from build123d import *

# Parameters (mm, degrees)
SKETCH_1_W               = 50
SKETCH_1_H               = 60
EXTRUDE_1_DEPTH          = 70
DRAFT_1_ANGLE            = 1.591
CUT_EXTRUDE_1_DEPTH      = 105.880884817
CUT_EXTRUDE_1_DEPTH_BACK = 105.880884817
SKETCH_8_R               = 30
SKETCH_9_R               = 29.988439116
CUT_EXTRUDE_2_DEPTH      = 93.836652593
SKETCH_10_W              = 61.388766385
SKETCH_10_H              = 50
CUT_EXTRUDE_3_DEPTH      = 93.836652759
SHELL_1_T                = -3
SKETCH_11_R              = 2.125
CUT_EXTRUDE_4_DEPTH      = 64.305956024


with BuildPart() as part:
    # 草圖1 → 填料-伸長1 (new body)
    with BuildSketch(Plane(origin=(0, 0, 0), x_dir=(1, 0, 0), z_dir=(0, 1, 0))):
        with Locations((25, 0)):
            Rectangle(SKETCH_1_W, SKETCH_1_H)
    extrude(amount=EXTRUDE_1_DEPTH)

    # 拔模1
    draft_1_faces = [part.faces().sort_by_distance(p)[0] for p in [
        (50, 35, 0),
        (25, 35, -30),
    ]]
    draft(draft_1_faces, Plane.ZX.offset(70), DRAFT_1_ANGLE)

    # 草圖8 → 除料-伸長1 (cut, two sides: drawn at the far end of the back side and taken through both)
    with BuildSketch(Plane(origin=(50, 70, -30), x_dir=(0.9996147856379402, 0.027743225206125616, 0.0007705771714084014), z_dir=(0.027753924659674706, -0.9992294227713525, -0.027753924659674706)).offset(-CUT_EXTRUDE_1_DEPTH_BACK)):
        Circle(SKETCH_8_R)
    extrude(amount=CUT_EXTRUDE_1_DEPTH + CUT_EXTRUDE_1_DEPTH_BACK, mode=Mode.SUBTRACT)

    # 草圖9 → 除料-伸長2 (cut, through all)
    with BuildSketch(Plane(origin=(0, 70, 0), x_dir=(1, 0, 0), z_dir=(0, 1, 0))):
        with Locations((50, -30)):
            Circle(SKETCH_9_R)
    extrude(amount=-CUT_EXTRUDE_2_DEPTH, mode=Mode.SUBTRACT)

    # 草圖10 → 除料-伸長3 (cut, through all)
    with BuildSketch(Plane.ZY):
        with Locations((-0.694383192, 45)):
            Rectangle(SKETCH_10_W, SKETCH_10_H)
    extrude(amount=-CUT_EXTRUDE_3_DEPTH, mode=Mode.SUBTRACT)

    # 薄殼1
    shell_1_openings = [part.faces().sort_by_distance(p)[0] for p in [
        (14.872442298, 20, -1.069608967),
        (10.828073147, 9.957245624, -31.667707178),
        (10.005780442, 10, 30),
        (0, 9.984986274, -0.833468336),
    ]]
    offset(amount=SHELL_1_T, openings=shell_1_openings, kind=Kind.INTERSECTION)

    # 草圖11 → 除料-伸長4 (cut, through all)
    with BuildSketch(Plane(origin=(0, 3, 0), x_dir=(1, 0, 0), z_dir=(0, 1, 0))):
        with Locations(Location((10, 15, 0), (0, 0, 270))):
            Circle(SKETCH_11_R)
        with Locations(Location((10, -15, 0), (0, 0, 90))):
            Circle(SKETCH_11_R)
    extrude(amount=-CUT_EXTRUDE_4_DEPTH, mode=Mode.SUBTRACT)


solid = part.part
Source: CAD feature listing. Evaluate the final solid. Frame: model axes, mm. Give positions to 0.01 mm unless a question says otherwise; leave off trailing zeros. Write each loop counter-clockwise with the first axis right and the second up, starting at its lowest first coordinate (ties: lowest second). Pieces come first, ordered by that corner, then holes. Notation, with made-up numbers: M 59,52.25 L 91,52.25 A15 ccw 91,73.25 Z; hole C 84.25,26.5 d5. An arc over 180 degrees is marked long. Return JSON: item names as keys, results as strings. Group by question number.
1) Cut plane A-A, the plane x = 10. Output: boundary loops of the cut face in (y, z) (3 decimals), plus the area to 3 significant figures.
2) Material intervals for line 1 along Y through (x, z) = (15, -8); line 2 along X through (y, z) = (1.2, 15) (3 decimals); line 3 along Z through (x, y) = (38.5, 10), sorted ascending. Write a range as [from, to].
3) Pull-direction query (X, two-part tool) for faces 1 (the face through (0, 1, -1)), 2 (the face through (11, 3, -1)), 3 (the face through (11.29, 1.52, 16.69)); classes: pulls with the +X half, pulls with the -X half, needs draft (parallel to the pull), parting line crosses it, or undercut.
4) Cut plane B-B, the plane z = 15.5. Output: boundary loops of the cut face in (x, y), plus the area to 3 significant figures.
5) Pin query (flat end, axial travel): P1, Ø5, axis at x = 10, z = 15, coming from the +Y side; P2, Ø6, axis at y = 9, z = -20.5, coming from the +X side; P3, Ø5, axis at y = 11, z = -18.5, coming from the +X side. Return the tip coordinate at first contact, or that it passes through.
Recorded:
{
 "1": {"outline": "M 0,-31.944 L 3,-31.861 L 3,-17.125 L 0,-17.125 Z; M 0,-12.875 L 3,-12.875 L 3,12.875 L 0,12.875 Z; M 0,17.125 L 3,17.125 L 3,30 L 0,30 Z", "area": "160 mm²"},
 "2": {"line 1": "y = [0, 3]", "line 2": "x = [0, 7.875], [12.125, 24.033]", "line 3": "z = [-4.69, -1.38], [-0.92, 2.3]"},
 "3": {"face 1": "pulls with the -X half", "face 2": "needs draft", "face 3": "undercut"},
 "4": {"outline": "M 0,0 L 7.93,0 L 7.93,3 L 0,3 Z; M 12.07,0 L 23.75,0 L 23.75,20 L 20.37,20 L 20.37,3 L 12.07,3 Z", "area": "116 mm²"},
 "5": {"P1": "stops at y = 3", "P2": "stops at x = 25.25", "P3": "stops at x = 26.02"}
}
